Can you work these out from the model? Positions are in its coordinate system, mm. Round coordinates to 2 decimals unless told otherwise and drop trailing zeros. Write each loop counter-clockwise with the first axis right and the second up, starting at its lowest first coordinate (ties: lowest second). Pieces come first, ordered by that corner, then holes. Notation, with made-up numbers: (-14.75, 31.25) -> (36.25, 31.25) arc R26 ccw to (36.25, 50.25) -> close; hole circle Ø1 at (45.25, -7.75). An arc over 180 degrees is marked (long way). Use CSV: the item, a comma, the result in double quotes.
```python
from build123d import *

# Parameters (mm, degrees)
SKETCH_1_W          = 100
SKETCH_1_H          = 80
EXTRUDE_1_DEPTH     = 10
SKETCH_3_R          = 2.6
CUT_EXTRUDE_2_DEPTH = 65.807406984
SKETCH_4_R          = 1.55
CUT_EXTRUDE_3_DEPTH = 65.807406984


with BuildPart() as part:
    # 草图1 → 凸台-拉伸1 (new body)
    with BuildSketch(Plane(origin=(0, 0, 0), x_dir=(1, 0, 0), z_dir=(0, 1, 0))):
        Rectangle(SKETCH_1_W, SKETCH_1_H)
    extrude(amount=EXTRUDE_1_DEPTH)

    # 草图3 → 切除-拉伸2 (cut, through all)
    with BuildSketch(Plane.XZ):
        with Locations(Location((40, 30, 0), (0, 0, 270))):
            Circle(SKETCH_3_R)
        with Locations(Location((40, 10, 0), (0, 0, 270))):
            Circle(SKETCH_3_R)
        with Locations(Location((-40, 30, 0), (0, 0, 270))):
            Circle(SKETCH_3_R)
        with Locations(Location((-40, 10, 0), (0, 0, 270))):
            Circle(SKETCH_3_R)
    extrude(amount=-CUT_EXTRUDE_2_DEPTH, mode=Mode.SUBTRACT)

    # 草图4 → 切除-拉伸3 (cut, through all)
    with BuildSketch(Plane(origin=(0, 10, 0), x_dir=(1, 0, 0), z_dir=(0, 1, 0))):
        with Locations(Location((14, 33.8, 0), (0, 0, 270))):
            Circle(SKETCH_4_R)
        with Locations(Location((14, 5.8, 0), (0, 0, 270))):
            Circle(SKETCH_4_R)
        with Locations(Location((-14, 33.8, 0), (0, 0, 270))):
            Circle(SKETCH_4_R)
        with Locations(Location((-14, 5.8, 0), (0, 0, 270))):
            Circle(SKETCH_4_R)
    extrude(amount=-CUT_EXTRUDE_3_DEPTH, mode=Mode.SUBTRACT)


solid = part.part
```
Q1. Will this pin go through, and if not, where does the flat tip stop? P1, Ø4, axis at x = -14, z = -5.8, coming from the +Y side.
Resolved:
P1,"stops at y = 10"
Q2. Suppose I cut it at B-B (x = 14). Write out the boundary of the cut face in (y, z).
Resolved:
outline,"(0, -40) -> (10, -40) -> (10, -35.35) -> (0, -35.35) -> close; (0, -32.25) -> (10, -32.25) -> (10, -7.35) -> (0, -7.35) -> close; (0, -4.25) -> (10, -4.25) -> (10, 40) -> (0, 40) -> close"
Q3. Suppose I cut it at A-A (z = 30). Write out the boundary of the cut face in (x, y), and give its area (3 significant figures).
Resolved:
outline,"(-50, 0) -> (-42.6, 0) -> (-42.6, 10) -> (-50, 10) -> close; (-37.4, 0) -> (37.4, 0) -> (37.4, 10) -> (-37.4, 10) -> close; (42.6, 0) -> (50, 0) -> (50, 10) -> (42.6, 10) -> close"
area,"896 mm^2"
Q4. Please list where these lines run through material, in increasing order: probe 1 along X at (y, z) = (7.25, 10); probe 2 along X at (y, z) = (3.5, -5.8).
Resolved:
probe 1,"x = -50 to -42.6, -37.4 to 37.4, 42.6 to 50"
probe 2,"x = -50 to -15.55, -12.45 to 12.45, 15.55 to 50"
Q5. If we mould it in two halves opening along Z, with no side actions, what happens to faces 1 (the face through (-1, 5, 40)), 2 (the face through (50, 5, 1)), 3 (the face through (15.537, 5.07, -6.002))? For each: released by +Z, released by -Z, zero draft, split by the parting line, or undercut.
Resolved:
face 1,"released by +Z"
face 2,"zero draft"
face 3,"undercut"
